Verification items for the finished model (mm, model axes). A direction names the side the tool comes from. Coordinates: 2 decimals unless noted, no trailing zeros. Order: outer loops, then holes, each group sorted by start corner. A loop starts at its lowest first (then second) coordinate and runs counter-clockwise, first axis right, second up. Notation, with made-up numbers: M 76.5,83 L 132.5,83 A12 cw 132.5,90 Z; hole C -17,89 d3. An arc over 180 degrees is marked long. Return JSON: item names as keys, results as strings. Group by question number.
Q1. Thickness scan on probe 1 along X at (y, z) = (-3, 36.5); probe 2 along Y at (x, z) = (-11.25, 43); probe 3 along Y at (x, z) = (14.25, 6). Record the ranges inside material, lowest first.
Q2. Go/stop test with a flat-tipped pin: pin 1 Ø3 at (y, z) = (0, 25) entering from -X. Record where the tip stops, or that it passes through.
Q3. Section check A-A, the plane x = 7.5. Enter the section's corners in (y, z), then the cut area to 3 significant figures.
Q4. Mould release check, pull along X, two halves, no side actions. Record for faces 1 (the face through (-14.877, -5, 25)), 2 (the face through (-5, -4.243, 25)), 3 (the face through (-13, -2.493, 25)): pulls with the +X half, pulls with the -X half, needs draft (parallel to the pull), parting line crosses it, or undercut.
Q5. Section check B-B, the plane y = 3. Enter the section's corners in (x, z), then the cut area to 3 significant figures.
Q6. Access from +Z, -Z, +X, -X, +Y, -Y to the whole of each face (thin tool, end or side, straight path). Record for faces 4 (the face through (8, -4.243, 25)), 5 (the face through (14, -2.493, 25)), 6 (the face through (0, 8.757, 25)).
from build123d import *

# Parameters (mm, degrees)
EXTRUDE_1_DEPTH = 50


with BuildPart() as part:
    # 草图1 → 凸台-拉伸1 (new body)
    with BuildSketch(Plane.XY):
        with BuildLine():
            Line((-11.577197952, 5.757012623), (0.822802048, 5.757012623))
            ThreePointArc((0.822802048, 5.757012623), (1.034934082, 5.669144657), (1.122802048, 5.457012623))
            Line((1.122802048, 5.457012623), (1.122802048, -3.942987377))
            ThreePointArc((1.122802048, -3.942987377), (1.034934082, -4.155119412), (0.822802048, -4.242987377))
            Line((0.822802048, -4.242987377), (-11.577197952, -4.242987377))
            ThreePointArc((-11.577197952, -4.242987377), (-11.789329987, -4.155119412), (-11.877197952, -3.942987377))
            Line((-11.877197952, -3.942987377), (-11.877197952, -2.792987377))
            ThreePointArc((-11.877197952, -2.792987377), (-11.965065918, -2.580855343), (-12.177197952, -2.492987377))
            Line((-12.177197952, -2.492987377), (-14.577197952, -2.492987377))
            ThreePointArc((-14.577197952, -2.492987377), (-14.789329987, -2.580855343), (-14.877197952, -2.792987377))
            Line((-14.877197952, -2.792987377), (-14.877197952, -6.942987377))
            ThreePointArc((-14.877197952, -6.942987377), (-14.789329987, -7.155119412), (-14.577197952, -7.242987377))
            Line((-14.577197952, -7.242987377), (14.822802048, -7.242987377))
            ThreePointArc((14.822802048, -7.242987377), (15.034934082, -7.155119412), (15.122802048, -6.942987377))
            Line((15.122802048, -6.942987377), (15.122802048, -2.792987377))
            ThreePointArc((15.122802048, -2.792987377), (15.034934082, -2.580855343), (14.822802048, -2.492987377))
            Line((14.822802048, -2.492987377), (12.422802048, -2.492987377))
            ThreePointArc((12.422802048, -2.492987377), (12.210670013, -2.580855343), (12.122802048, -2.792987377))
            Line((12.122802048, -2.792987377), (12.122802048, -3.942987377))
            ThreePointArc((12.122802048, -3.942987377), (12.034934082, -4.155119412), (11.822802048, -4.242987377))
            Line((11.822802048, -4.242987377), (4.422802048, -4.242987377))
            ThreePointArc((4.422802048, -4.242987377), (4.210670013, -4.155119412), (4.122802048, -3.942987377))
            Line((4.122802048, -3.942987377), (4.122802048, 5.457012623))
            ThreePointArc((4.122802048, 5.457012623), (4.210670013, 5.669144657), (4.422802048, 5.757012623))
            Line((4.422802048, 5.757012623), (11.822802048, 5.757012623))
            ThreePointArc((11.822802048, 5.757012623), (12.034934082, 5.669144657), (12.122802048, 5.457012623))
            Line((12.122802048, 5.457012623), (12.122802048, 4.307012623))
            ThreePointArc((12.122802048, 4.307012623), (12.210670013, 4.094880588), (12.422802048, 4.007012623))
            Line((12.422802048, 4.007012623), (14.822802048, 4.007012623))
            ThreePointArc((14.822802048, 4.007012623), (15.034934082, 4.094880588), (15.122802048, 4.307012623))
            Line((15.122802048, 4.307012623), (15.122802048, 8.457012623))
            ThreePointArc((15.122802048, 8.457012623), (15.034934082, 8.669144657), (14.822802048, 8.757012623))
            Line((14.822802048, 8.757012623), (-14.577197952, 8.757012623))
            ThreePointArc((-14.577197952, 8.757012623), (-14.789329987, 8.669144657), (-14.877197952, 8.457012623))
            Line((-14.877197952, 8.457012623), (-14.877197952, 4.307012623))
            ThreePointArc((-14.877197952, 4.307012623), (-14.789329987, 4.094880588), (-14.577197952, 4.007012623))
            Line((-14.577197952, 4.007012623), (-12.177197952, 4.007012623))
            ThreePointArc((-12.177197952, 4.007012623), (-11.965065918, 4.094880588), (-11.877197952, 4.307012623))
            Line((-11.877197952, 4.307012623), (-11.877197952, 5.457012623))
            ThreePointArc((-11.877197952, 5.457012623), (-11.789329987, 5.669144657), (-11.577197952, 5.757012623))
        make_face()
    extrude(amount=EXTRUDE_1_DEPTH)


solid = part.part
Numbers:
{
 "1": {"probe 1": "x = -14.88 to -11.88, 1.12 to 4.12, 12.12 to 15.12", "probe 2": "y = -7.24 to -4.24, 5.76 to 8.76", "probe 3": "y = -7.24 to -2.49, 4.01 to 8.76"},
 "2": {"pin 1": "stops at x = 1.12"},
 "3": {"outline": "M -7.24,0 L -4.24,0 L -4.24,50 L -7.24,50 Z; M 5.76,0 L 8.76,0 L 8.76,50 L 5.76,50 Z", "area": "300 mm2"},
 "4": {"face 1": "pulls with the -X half", "face 2": "undercut", "face 3": "needs draft"},
 "5": {"outline": "M 1.12,0 L 4.12,0 L 4.12,50 L 1.12,50 Z", "area": "150 mm2"},
 "6": {"face 4": "+Z, -Z", "face 5": "+Z, -Z, +X", "face 6": "+Z, -Z, +X, -X, +Y"}
}
